Could you check a few things on this model? Use its own coordinates, in mm. Face numbers are marked on the shaded views. A direction names the side the tool comes from. Give positions to 0.01 mm unless a question says otherwise; leave off trailing zeros. Write each loop counter-clockwise with the first axis right and the second up, starting at its lowest first coordinate (ties: lowest second). Pieces come first, ordered by that corner, then holes. Notation, with made-up numbers: (-26, -1) -> (13, -1) arc R36 ccw to (13, 34) -> close; hole circle Ø1 at (42.25, 66.25). An arc over 180 degrees is marked (long way). One line per question, with ' | ' between items.
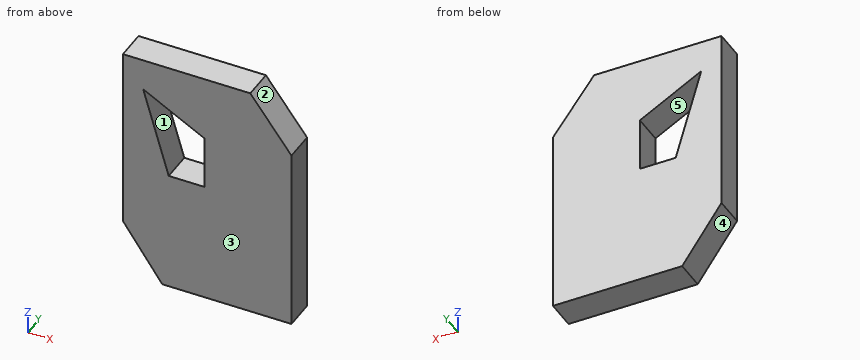
from build123d import *

# Parameters (mm, degrees)
F0_W     = 106.714278
F0_H     = 155.109674
F1_DEPTH = 25.4


with BuildPart() as f1:
    # F0 (on Front) → F1 (new body)
    with BuildSketch(Plane.XZ):
        Polygon((87.841675, -47.520965), (53.357139, 0), (-53.357139, 0), (-20.406917, -47.520965), align=None)
        with Locations((0, 77.554837)):
            Rectangle(F0_W, F0_H)
        Polygon((14.997154, 55.01838), (-14.997154, 55.01838), (-36.390718, 128.240824), (14.997154, 100.091293), align=None, mode=Mode.SUBTRACT)
        Polygon((53.357139, 155.109674), (53.357139, 0), (87.841675, -47.520965), (87.841675, 108.981639), align=None)
    extrude(amount=F1_DEPTH)


solid = f1.part
Q1. Imagine slicing it at C-C on x = -7. Please give me the cut outline in (y, z), and give its area (3 significant figures).
Answer below:
outline: (-25.4, -47.52) -> (0, -47.52) -> (0, 55.02) -> (-25.4, 55.02) -> close; (-25.4, 112.14) -> (0, 112.14) -> (0, 155.11) -> (-25.4, 155.11) -> close | area: 3,700 mm^2
Q2. If I drill on line 1 along X through (y, z) = (-10, 92); line 2 along Z through (x, y) = (-8, -11); line 3 along X through (y, z) = (-6, 120.5), over which ranges is the centre line in solid material (lowest first)?
Answer below:
line 1: x = -53.36 to -25.8, 15 to 87.84 | line 2: z = -47.52 to 55.02, 112.69 to 155.11 | line 3: x = -53.36 to -34.13, -22.26 to 79.23
Q3. Imagine slicing it at A-A on y = -15. Please give me the cut outline in (x, z), and give its area (3 significant figures).
Answer below:
outline: (-53.36, 0) -> (-20.41, -47.52) -> (87.84, -47.52) -> (87.84, 108.98) -> (53.36, 155.11) -> (-53.36, 155.11) -> close; hole (-36.39, 128.24) -> (-15, 55.02) -> (15, 55.02) -> (15, 100.09) -> close | area: 24,800 mm^2
Q4. Imagine slicing it at B-B on z = 93. Please give me the cut outline in (x, y).
Answer below:
outline: (-53.36, -25.4) -> (-26.09, -25.4) -> (-26.09, 0) -> (-53.36, 0) -> close; (15, -25.4) -> (87.84, -25.4) -> (87.84, 0) -> (15, 0) -> close
Q5. If we mould it in two halves opening along Z, with no side actions, what happens to the marked faces 3, 4 and 5? For each: +Z half, -Z half, draft (parallel to the pull), parting line (faces both ways), or undercut.
Answer below:
face 3: draft | face 4: -Z half | face 5: undercut
Q6. Imagine slicing it at D-D on z = -21. Please give me the cut outline in (x, y).
Answer below:
outline: (-38.8, -25.4) -> (87.84, -25.4) -> (87.84, 0) -> (-38.8, 0) -> close
Q7. On a 3-axis mill with a long thin cutter (end or side, diameter ignored), from which of +Z, -Z, +X, -X, +Y, -Y can I reach the whole of each face in a straight line? I mean the marked faces 1 and 2. Say none if no direction works.
Answer below:
face 1: +Y, -Y | face 2: +Z, +X, +Y, -Y
Q8. Will these pins go through, and if not, where does the flat tip stop? pin 1 (1.5 mm diameter, centred on x = 49, z = 54.5, fed in from +Y); pin 2 (10 mm diameter, centred on y = -19, z = 118.5, fed in from +X).
Answer below:
pin 1: stops at y = 0 | pin 2: stops at x = 84.46
